The model under review builds one solid part; all positions refer to its coordinate system, in mm. Face numbers are marked on the shaded views. Give positions to 0.01 mm unless a question says otherwise; leave off trailing zeros. Order: outer loops, then holes, each group sorted by start corner. A loop starts at its lowest first (then second) coordinate and runs counter-clockwise, first axis right, second up.
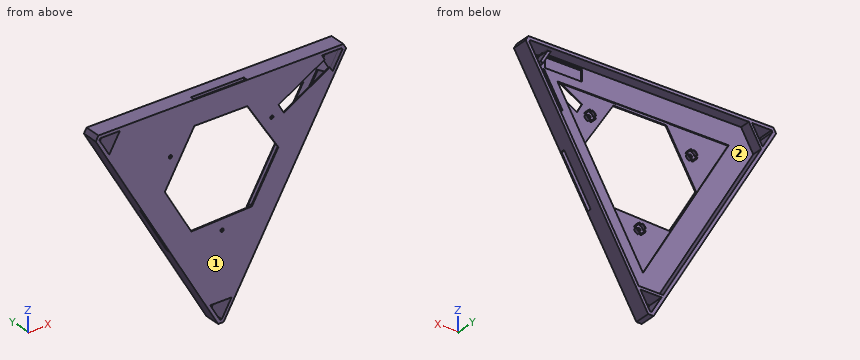
```python
from build123d import *

# Parameters (mm, degrees)
SKETCH1_W                = 34.714871787
SKETCH1_H                = 10.923666426
BOSS_EXTRUDE1_DEPTH      = 1
BOSS_EXTRUDE2_DEPTH      = 11
BOSS_EXTRUDE3_DEPTH      = 5
BOSS_EXTRUDE3_DEPTH_BACK = 3
SKETCH3_W                = 50
SKETCH3_H                = 7
CUT_EXTRUDE3_DEPTH       = 25
SKETCH5_W                = 50
SKETCH5_H                = 7
CUT_EXTRUDE4_DEPTH       = 25
SKETCH6_W                = 50
SKETCH6_H                = 7
CUT_EXTRUDE5_DEPTH       = 25
SKETCH8_R                = 1.5
BOSS_EXTRUDE5_DEPTH      = 1
BOSS_EXTRUDE10_DEPTH     = 3


with BuildPart() as part:
    # Sketch1 → Boss-Extrude1 (new body)
    with BuildSketch(Plane(origin=(0, 0, 0), x_dir=(1, 0, 0), z_dir=(0, 1, 0))):
        Polygon((243.304219775, -116.484791865), (254.809280577, -136.408896137), (442.602090749, -136.409305398), (444.621046679, -132.925433224), (441.749040748, -132.925433224), (449.516726724, -119.471406458), (450.964695298, -121.978953123), (452.699916622, -118.984688018), (358.778179036, 43.666038065), (335.767496284, 43.666038065), align=None)
        with Locations((422.370878913, -129.522754792)):
            Rectangle(SKETCH1_W, SKETCH1_H, mode=Mode.SUBTRACT)
        Polygon((423.190377512, -92.577472767), (432.651287025, -87.114324326), (450.119365975, -117.364996826), (440.658456462, -122.828145267), align=None, mode=Mode.SUBTRACT)
        Polygon((428.113670919, -116.417164681), (266.439108268, -116.428009237), (347.273609729, 23.609230821), align=None, mode=Mode.SUBTRACT)
    extrude(amount=BOSS_EXTRUDE1_DEPTH)

    # Sketch1_9 → Boss-Extrude2 (add)
    # profile 1 of 2: a face of its own
    with BuildSketch(Plane(origin=(0, 0, 0), x_dir=(1, 0, 0), z_dir=(0, 1, 0))):
        Polygon((229.159432548, -134.984249184), (231.716666588, -139.412373829), (462.829865412, -139.412373829), (465.38624875, -134.984588004), (349.829542096, 65.165499075), (344.716133219, 65.165499075), align=None)
        Polygon((251.922647989, -136.409305399), (233.446303401, -136.408896138), (232.62355396, -134.984217357), (241.860901689, -118.984688018), align=None, mode=Mode.SUBTRACT)
        Polygon((442.602090749, -136.409305398), (254.809280577, -136.408896137), (243.304219775, -116.484791865), (335.767496284, 43.666038065), (358.778179036, 43.666038065), (461.938967958, -134.984588006), (461.116393749, -136.409305398), align=None, mode=Mode.SUBTRACT)
        Polygon((348.096628302, 62.164013367), (357.334800991, 46.166038067), (337.210874326, 46.166038067), (346.44844193, 62.165948237), align=None, mode=Mode.SUBTRACT)
    # profile 2 of 2: a face of its own
    with BuildSketch(Plane(origin=(0, 0, 0), x_dir=(1, 0, 0), z_dir=(0, 1, 0))):
        Polygon((441.749040748, -132.925433224), (444.621046679, -132.925433224), (450.964695298, -121.978953123), (449.516726724, -119.471406458), align=None)
    extrude(amount=BOSS_EXTRUDE2_DEPTH)

    # Sketch1_10 → Boss-Extrude3 (add, two sides: drawn at the far end of the back side and taken through both)
    with BuildSketch(Plane(origin=(0, 0, 0), x_dir=(1, 0, 0), z_dir=(0, 1, 0)).offset(-BOSS_EXTRUDE3_DEPTH_BACK)):
        Polygon((229.159432548, -134.984249184), (231.716666588, -139.412373829), (462.829865412, -139.412373829), (465.38624875, -134.984588004), (349.829542096, 65.165499075), (344.716133219, 65.165499075), align=None)
        Polygon((251.922647989, -136.409305399), (233.446303401, -136.408896138), (232.62355396, -134.984217357), (241.860901689, -118.984688018), align=None, mode=Mode.SUBTRACT)
        Polygon((442.602090749, -136.409305398), (254.809280577, -136.408896137), (243.304219775, -116.484791865), (335.767496284, 43.666038065), (358.778179036, 43.666038065), (452.699916622, -118.984688018), (461.938967958, -134.984588006), (461.116393749, -136.409305398), align=None, mode=Mode.SUBTRACT)
        Polygon((348.096628302, 62.164013367), (357.334800991, 46.166038067), (337.210874326, 46.166038067), (346.44844193, 62.165948237), align=None, mode=Mode.SUBTRACT)
    extrude(amount=BOSS_EXTRUDE3_DEPTH + BOSS_EXTRUDE3_DEPTH_BACK)

    # Sketch3 → Cut-Extrude3 (cut)
    with BuildSketch(Plane(origin=(290.589645397, 0, -167.772009994), x_dir=(-0.49999999999998745, 0, -0.8660254037844459), z_dir=(0.8660254037844459, 0, -0.49999999999998745))):
        with Locations((-236.592990632, -3)):
            Rectangle(SKETCH3_W, SKETCH3_H)
    extrude(amount=-CUT_EXTRUDE3_DEPTH, mode=Mode.SUBTRACT)

    # Sketch5 → Cut-Extrude4 (cut)
    with BuildSketch(Plane.XY.offset(139.412373829)):
        with Locations((347.273266, -3)):
            Rectangle(SKETCH5_W, SKETCH5_H)
    extrude(amount=-CUT_EXTRUDE4_DEPTH, mode=Mode.SUBTRACT)

    # Sketch6 → Cut-Extrude5 (cut)
    with BuildSketch(Plane(origin=(230.319375798, 0, 132.975171837), x_dir=(-0.5000006154012504, 0, 0.8660250484820695), z_dir=(-0.8660250484820695, 0, -0.5000006154012504))):
        with Locations((-113.236674799, -3)):
            Rectangle(SKETCH6_W, SKETCH6_H)
    extrude(amount=-CUT_EXTRUDE5_DEPTH, mode=Mode.SUBTRACT)

    # Sketch8 → Boss-Extrude5 (add)
    with BuildSketch(Plane.XZ.offset(3)):
        Polygon((349.829542096, -65.165499075), (465.38624875, 134.984588004), (462.829865412, 139.412373829), (231.716666588, 139.412373829), (229.159432548, 134.984249184), (344.716133219, -65.165499075), align=None)
        with Locations(Location((395.323540807, 98.692824234, 0), (0, 0, 270))):
            Circle(SKETCH8_R, mode=Mode.SUBTRACT)
        with Locations(Location((348.301285091, 15.863526629, 0), (0, 0, 270))):
            Circle(SKETCH8_R, mode=Mode.SUBTRACT)
        with Locations(Location((299.654911442, 97.24168178, 0), (0, 0, 270))):
            Circle(SKETCH8_R, mode=Mode.SUBTRACT)
        Polygon((450.14703547, 123.280701064), (452.699916622, 118.984688018), (461.938967958, 134.984588006), (461.116393749, 136.409305398), (442.602090749, 136.409305398), (445.226665069, 131.986443715), (401.697951811, 107.384591709), (406.618322213, 98.678849058), align=None, mode=Mode.SUBTRACT)
        Polygon((322.273266, 116.42426408), (294.358218631, 68.061097964), (319.354499367, 24.757680453), (376.473657316, 26.969372806), (401.47267951, 70.271207531), (372.273266, 116.420910257), align=None, mode=Mode.SUBTRACT)
        Polygon((233.446303401, 136.408896138), (251.922647989, 136.409305399), (241.860901689, 118.984688018), (232.62355396, 134.984217357), align=None, mode=Mode.SUBTRACT)
        Polygon((337.210874326, -46.166038067), (357.334800991, -46.166038067), (348.096628302, -62.164013367), (346.44844193, -62.165948237), align=None, mode=Mode.SUBTRACT)
    extrude(amount=BOSS_EXTRUDE5_DEPTH)

    # Sketch12 → Boss-Extrude10 (add)
    with BuildSketch(Plane(origin=(0, -3, 0), x_dir=(1, 0, 0), z_dir=(0, 1, 0))):
        with BuildLine():
            Line((347.417900211, -11.962292061), (347.307477101, -11.47463774))
            ThreePointArc((347.307477101, -11.47463774), (345.119304576, -12.681546114), (343.912396202, -14.869718639))
            Line((343.912396203, -14.869718639), (344.400050524, -14.980141749))
            ThreePointArc((344.400050523, -14.980141749), (345.472857967, -13.035099504), (347.417900211, -11.962292061))
        make_face()
        with BuildLine():
            ThreePointArc((352.690173981, -14.869718639), (351.483265607, -12.681546114), (349.295093082, -11.47463774))
            Line((349.295093081, -11.47463774), (349.184669971, -11.962292061))
            ThreePointArc((349.184669972, -11.962292061), (351.129712216, -13.035099504), (352.20251966, -14.980141749))
            Line((352.202519659, -14.980141749), (352.69017398, -14.869718639))
        make_face()
        with BuildLine():
            ThreePointArc((349.295093082, -20.252415518), (351.483265607, -19.045507145), (352.690173981, -16.857334619))
            Line((352.69017398, -16.857334619), (352.202519659, -16.746911509))
            ThreePointArc((352.20251966, -16.746911509), (351.129712216, -18.691953754), (349.184669972, -19.764761197))
            Line((349.184669971, -19.764761197), (349.295093081, -20.252415518))
        make_face()
        with BuildLine():
            Line((344.400050524, -16.746911509), (343.912396203, -16.857334619))
            ThreePointArc((343.912396202, -16.857334619), (345.119304576, -19.045507145), (347.307477101, -20.252415518))
            Line((347.307477101, -20.252415518), (347.417900211, -19.764761197))
            ThreePointArc((347.417900211, -19.764761197), (345.472857967, -18.691953754), (344.400050523, -16.746911509))
        make_face()
        with BuildLine():
            Line((394.440155927, -94.791589666), (394.329732817, -94.303935345))
            ThreePointArc((394.329732817, -94.303935345), (392.141560292, -95.510843718), (390.934651918, -97.699016244))
            Line((390.934651918, -97.699016244), (391.4247896, -97.798542945))
            ThreePointArc((391.4247896, -97.798542945), (392.499067689, -95.860448622), (394.440155927, -94.791589666))
        make_face()
        with BuildLine():
            ThreePointArc((399.712429696, -97.699016244), (398.505521323, -95.510843718), (396.317348797, -94.303935345))
            Line((396.317348797, -94.303935345), (396.206925687, -94.791589666))
            ThreePointArc((396.206925687, -94.791589666), (398.151967932, -95.864397109), (399.224775375, -97.809439354))
            Line((399.224775375, -97.809439354), (399.712429696, -97.699016244))
        make_face()
        with BuildLine():
            ThreePointArc((396.317348797, -103.081713123), (398.505521323, -101.874804749), (399.712429696, -99.686632224))
            Line((399.712429696, -99.686632224), (399.224775375, -99.576209114))
            ThreePointArc((399.224775375, -99.576209114), (398.151967932, -101.521251358), (396.206925687, -102.594058802))
            Line((396.206925687, -102.594058801), (396.317348797, -103.081713122))
        make_face()
        with BuildLine():
            Line((391.422306239, -99.576209114), (390.934651918, -99.686632224))
            ThreePointArc((390.934651918, -99.686632224), (392.141560292, -101.874804749), (394.329732817, -103.081713123))
            Line((394.329732817, -103.081713122), (394.440155927, -102.594058801))
            ThreePointArc((394.440155927, -102.594058802), (392.495113682, -101.521251358), (391.422306239, -99.576209114))
        make_face()
        with BuildLine():
            ThreePointArc((298.661103452, -92.852792892), (296.472930927, -94.059701265), (295.266022553, -96.24787379))
            Line((295.266022553, -96.24787379), (295.753676874, -96.3582969))
            ThreePointArc((295.753676874, -96.3582969), (296.826484317, -94.413254656), (298.771526562, -93.340447213))
            Line((298.771526562, -93.340447212), (298.661103452, -92.852792891))
        make_face()
        with BuildLine():
            ThreePointArc((304.04380033, -96.24787379), (302.836891957, -94.059701265), (300.648719432, -92.852792892))
            Line((300.648719432, -92.852792891), (300.538296322, -93.340447212))
            ThreePointArc((300.538296322, -93.340447213), (302.483338566, -94.413254656), (303.55614601, -96.3582969))
            Line((303.55614601, -96.3582969), (304.043800331, -96.24787379))
        make_face()
        with BuildLine():
            Line((300.538296322, -101.142916348), (300.648719432, -101.630570669))
            ThreePointArc((300.648719432, -101.630570669), (302.836891957, -100.423662295), (304.04380033, -98.23548977))
            Line((304.043800331, -98.23548977), (303.55614601, -98.12506666))
            ThreePointArc((303.55614601, -98.12506666), (302.483338566, -100.070108905), (300.538296322, -101.142916348))
        make_face()
        with BuildLine():
            Line((295.753676874, -98.12506666), (295.266022553, -98.23548977))
            ThreePointArc((295.266022553, -98.23548977), (296.472930927, -100.423662295), (298.661103452, -101.630570669))
            Line((298.661103452, -101.630570669), (298.771526562, -101.142916348))
            ThreePointArc((298.771526562, -101.142916348), (296.826484317, -100.070108905), (295.753676874, -98.12506666))
        make_face()
    extrude(amount=BOSS_EXTRUDE10_DEPTH)


solid = part.part
```
1. Take a section at A-A (y = 5.25). Write out the cut boundary in (x, z).
2. Take a section at C-C (z = 41.5). Write out the cut boundary in (x, y).
3. Take a section at D-D (z = 84). Write out the cut boundary in (x, y).
4. Insertion check: pin 1 (1 mm diameter, centred on x = 331, y = 5, fed in from -Z); pin 2 (12 mm diameter, centred on x = 423, z = 90, fed in from +Y); pin 3 (0.5 mm diameter, centred on x = 358, y = -3.5, fed in from -Z). Each pin has a flat end and moves straight along its axis. Give the tip position at first contact, or say it passes through.
5. Take a section at B-B (x = 387.5). Write out the cut boundary in (y, z), and give its area (3 significant figures).
6. Draft analysis for pull direction Z (two halves, no side actions). For the marked faces 1 and 2, state which applies: pulls with the +Z half, pulls with the -Z half, needs draft (parallel to the pull), parting line crosses it, or undercut.
7. To check wall thickness, follow line 1 (Y direction, x = 296, z = 38); line 2 (Z direction, x = 284.5, y = -1.25); line 3 (Z direction, x = 384.5, y = 2.75). State the ranges of each line that lie inside material, in increasing order.
Answer:
1. outline: (229.16, 134.98) - (344.72, -65.17) - (349.83, -65.17) - (465.39, 134.98) - (462.83, 139.41) - (231.72, 139.41) - close; (441.75, 132.93) - (449.52, 119.47) - (450.96, 121.98) - (444.62, 132.93) - close; hole (232.62, 134.98) - (241.86, 118.98) - (251.92, 136.41) - (233.45, 136.41) - close; hole (243.3, 116.48) - (335.77, -43.67) - (358.78, -43.67) - (461.94, 134.98) - (461.12, 136.41) - (442.6, 136.41) - (254.81, 136.41) - close; hole (337.21, -46.17) - (346.45, -62.17) - (348.1, -62.16) - (357.33, -46.17) - close
2. outline: (283.13, -4) - (309.69, -4) - (309.69, -3) - (283.13, -3) - close; (283.13, 0.5) - (309.69, 0.5) - (309.69, 1) - (286.6, 1) - (286.6, 11) - (283.13, 11) - close; (384.86, -4) - (411.41, -4) - (411.41, -3) - (384.86, -3) - close; (384.86, 0.5) - (411.41, 0.5) - (411.41, 11) - (407.96, 11) - (407.96, 1) - (384.86, 1) - close
3. outline: (258.6, -4) - (303.56, -4) - (303.56, -3) - (262.06, -3) - (262.06, 0) - (285.16, 0) - (285.16, 1) - (262.06, 1) - (262.06, 11) - (258.6, 11) - close; (392.79, -4) - (435.95, -4) - (435.95, 11) - (432.5, 11) - (432.5, 1) - (409.4, 1) - (409.4, 0) - (432.5, 0) - (432.5, -3) - (392.79, -3) - close
4. pin 1: stops at z = -42.27
4. pin 2: stops at y = 1
4. pin 3: stops at z = -51.45
5. outline: (-4, 0.08) - (11, 0.08) - (11, 6.07) - (1, 6.07) - (1, 46.07) - (0.5, 46.07) - (0.5, 20.6) - (0, 20.6) - (0, 6.07) - (-3, 6.07) - (-3, 46.07) - (-4, 46.07) - close; (-4, 92.36) - (-3, 92.36) - (-3, 136.41) - (0, 136.41) - (0, 116.42) - (1, 116.42) - (1, 136.41) - (11, 136.41) - (11, 139.41) - (-4, 139.41) - close
5. area: 266 mm2
6. face 1: needs draft
6. face 2: undercut
7. line 1: y = -4 to -3, 0.5 to 1
7. line 2: z = 136.41 to 139.41
7. line 3: z = -5.11 to 0.88, 136.41 to 139.41
